```python
from build123d import *

# Parameters (mm, degrees)
F0_R        = 1.6
F0_R_2      = 11.2
F0_W        = 24
F0_H        = 13
F1_DEPTH    = 4
F2_W        = 24
F2_H        = 13
F3_DEPTH    = 40
F4_T4_DEPTH = 4
F4_T9_DEPTH = 4
F5_SIZE     = 8.99999
F6_R        = 2.1
F7_DEPTH    = 25
F6_R_2      = 4
F8_DEPTH    = 6
F9_SIZE     = 5


# Not quite as in the source:
# - a fillet or chamfer that OpenCascade refuses, or shapes differently, is made with other operations: its cross-section is extruded or revolved along the edge and cut away or added
# - a fillet or chamfer is up to 0.001 mm smaller than in the source, because OpenCascade refuses the exact size


with BuildPart() as f1:
    # F0 (on Top) → F1 (new body)
    with BuildSketch(Plane.XY):
        Polygon((12, -21), (21, -21), (21, 21), (-21, 21), (-21, -21), (-12, -21), align=None)
        with Locations((-15.5, -15.5)):
            Circle(F0_R, mode=Mode.SUBTRACT)
        with Locations((15.5, -15.5)):
            Circle(F0_R, mode=Mode.SUBTRACT)
        with Locations((-15.5, 15.5)):
            Circle(F0_R, mode=Mode.SUBTRACT)
        Circle(F0_R_2, mode=Mode.SUBTRACT)
        with Locations((15.5, 15.5)):
            Circle(F0_R, mode=Mode.SUBTRACT)
        with Locations((0, -27.5)):
            Rectangle(F0_W, F0_H)
    extrude(amount=F1_DEPTH)

    # F2 (on face) → F3 (join)
    with BuildSketch(Plane.XY.offset(4)):
        with Locations((0, -27.5)):
            Rectangle(F2_W, F2_H)
    extrude(amount=F3_DEPTH)

    # F4: chamfer of 13 on 2 edges, made by hand


with BuildPart() as f4_tool2:
    # F4_s3 → F4_t4 (new body)
    with BuildSketch(Plane.XY):
        Polygon((25, -21), (12, -34), (12, -21), align=None)
    extrude(amount=F4_T4_DEPTH)

    split(bisect_by=Plane.YZ.offset(21), keep=Keep.BOTTOM)


with BuildPart() as f1_1:
    add(f1.part)

    # F4_t1: union F4_tool2
    add(f4_tool2.part)


with BuildPart() as f4_tool7:
    # F4_s8 → F4_t9 (new body)
    with BuildSketch(Plane.XY):
        Polygon((-25, -21), (-12, -34), (-12, -21), align=None)
    extrude(amount=F4_T9_DEPTH)

    split(bisect_by=Plane.YZ.offset(-21), keep=Keep.TOP)


with BuildPart() as f1_2:
    add(f1_1.part)

    # F4_t6: union F4_tool7
    add(f4_tool7.part)

    # F5 (size 9 in the source; OpenCascade refuses exactly that, so slightly less here)
    f5_edges = [f1_2.edges().sort_by_distance(p)[0] for p in [
        (12, -27.5, 4),
        (-12, -27.5, 4),
    ]]
    chamfer(f5_edges, length=F5_SIZE)

    # F6 (on face) → F7 (cut)
    with BuildSketch(Plane(origin=(0, -21, 0), x_dir=(-1, 0, 0), z_dir=(0, 1, 0))):
        with Locations((0, 34)):
            Circle(F6_R)
        with Locations((0, 12)):
            Circle(F6_R)
    extrude(amount=-F7_DEPTH, mode=Mode.SUBTRACT)

    # F6 (on face) → F8 (cut)
    with BuildSketch(Plane(origin=(0, -21, 0), x_dir=(-1, 0, 0), z_dir=(0, 1, 0))):
        with Locations((0, 34)):
            Circle(F6_R_2)
        with Locations((0, 34)):
            Circle(F6_R, mode=Mode.SUBTRACT)
        with Locations((0, 12)):
            Circle(F6_R_2)
        with Locations((0, 12)):
            Circle(F6_R, mode=Mode.SUBTRACT)
    extrude(amount=-F8_DEPTH, mode=Mode.SUBTRACT)

    # F9
    f9_edges = [f1_2.edges().sort_by_distance(p)[0] for p in [
        (21, 21, 2),
        (-21, 21, 2),
    ]]
    chamfer(f9_edges, length=F9_SIZE)


solid = f1_2.part
```
Work out the finished part from the listing and answer in its coordinate system (mm). A direction names the side the tool comes from. Give positions to 0.01 mm unless a question says otherwise; leave off trailing zeros. Order: outer loops, then holes, each group sorted by start corner. A loop starts at its lowest first (then second) coordinate and runs counter-clockwise, first axis right, second up. Notation, with made-up numbers: (78, 33) -> (137, 33) arc R31 ccw to (137, 66) -> close; hole circle Ø11 at (-12.5, 24). An arc over 180 degrees is marked (long way). Answer as CSV lines item,"result". Start each with the question number.
(1) Section B-B, the plane y = -15.5 is taken. Write down the section's boundary in (x, z).
(2) Consider line 1 along Z through (x, y) = (0, -25); line 2 along Y through (x, z) = (-15.5, 1.8); line 3 along Z through (x, y) = (-17, 3.5). Determine where each line is inside the solid, lowest interval first.
(3) For a pull along Z with two mould halves and no side action, classify faces 4 (the cylindrical face through (0.273, -30.451, 14.082)), 5 (the flat face through (-18, 19, 2)), 6 (the flat face through (0, -12, 0)), 7 (the cylindrical face through (0.46, -30.45, 31.95)) as released by +Z, released by -Z, zero draft, split by the parting line, or undercut.
(4) Section C-C, the plane x = -15 is taken. Write down the section's boundary in (y, z), plus the area to 3 significant figures.
(5) Which of the six approach directions +Z, -Z, +X, -X, +Y, -Y give full straight-line access (tool end or side, diameter ignored) to faces 1 (the flat face through (-12, -28, 28)), 2 (the cylindrical face through (0.521, -23.958, 15.966)), 3 (the flat face through (-10, -7, 4))?
(6) Each of these flat-tipped pins is pushed along its axis until it touches: pin 1 Ø2.5 at (x, z) = (1, 12) entering from +Y; pin 2 Ø4 at (y, z) = (-28.5, 22) entering from +X; pin 3 Ø8 at (x, y) = (-5, -11.5) entering from +Z; pin 4 Ø2.5 at (x, z) = (0, 34) entering from -Y. Where does it stop, or does it pass through?
(7) Section A-A, the plane x = 0 is taken. Write down the section's boundary in (y, z).
(8) Section D-D, the plane y = 0 is taken. Write down the section's boundary in (x, z).
Entries:
1,outline,"(-21, 0) -> (-17.1, 0) -> (-17.1, 4) -> (-21, 4) -> close; (-13.9, 0) -> (13.9, 0) -> (13.9, 4) -> (-13.9, 4) -> close; (17.1, 0) -> (21, 0) -> (21, 4) -> (17.1, 4) -> close"
2,line 1,"0 to 8, 16 to 30, 38 to 44"
2,line 2,"-30.5 to -17.1, -13.9 to 13.9, 17.1 to 21"
2,line 3,"0 to 4"
3,face 4,"undercut"
3,face 5,"zero draft"
3,face 6,"released by -Z"
3,face 7,"undercut"
4,outline,"(-31, 0) -> (-17.02, 0) -> (-17.02, 4) -> (-21, 4) -> (-21, 10) -> (-31, 10) -> close; (-13.98, 0) -> (13.98, 0) -> (13.98, 4) -> (-13.98, 4) -> close; (17.02, 0) -> (21, 0) -> (21, 4) -> (17.02, 4) -> close"
4,area,"244 mm²"
5,face 1,"+Z, -X, +Y, -Y"
5,face 2,"+Y"
5,face 3,"+Z, +X, -X, +Y"
6,pin 1,"y = -27"
6,pin 2,"x = 12"
6,pin 3,"z = 4"
6,pin 4,"through"
7,outline,"(-34, 0) -> (-11.2, 0) -> (-11.2, 4) -> (-21, 4) -> (-21, 8) -> (-27, 8) -> (-27, 9.9) -> (-34, 9.9) -> close; (-34, 14.1) -> (-27, 14.1) -> (-27, 16) -> (-21, 16) -> (-21, 30) -> (-27, 30) -> (-27, 31.9) -> (-34, 31.9) -> close; (-34, 36.1) -> (-27, 36.1) -> (-27, 38) -> (-21, 38) -> (-21, 44) -> (-34, 44) -> close; (11.2, 0) -> (21, 0) -> (21, 4) -> (11.2, 4) -> close"
8,outline,"(-21, 0) -> (-11.2, 0) -> (-11.2, 4) -> (-21, 4) -> close; (11.2, 0) -> (21, 0) -> (21, 4) -> (11.2, 4) -> close"
